```python
from build123d import *

# Parameters (mm, degrees)
SKETCH1_W           = 23
SKETCH1_H           = 12
BOSS_EXTRUDE1_DEPTH = 22
SKETCH2_W           = 32
SKETCH2_H           = 12
BOSS_EXTRUDE2_DEPTH = 2
CUT_EXTRUDE1_DEPTH  = 5
SKETCH3_W           = 23
SKETCH3_H           = 12
BOSS_EXTRUDE4_DEPTH = 4
BOSS_EXTRUDE5_DEPTH = 4
SKETCH6_R           = 2.5
SKETCH6_R_2         = 2.25
BOSS_EXTRUDE6_DEPTH = 2
CUT_EXTRUDE2_START  = -4
SKETCH7_R           = 2.25
CUT_EXTRUDE2_DEPTH  = 4
FILLET4_R           = 0.5
SKETCH8_R           = 2.25
BOSS_EXTRUDE7_DEPTH = 1
SKETCH9_R           = 0.75
BOSS_EXTRUDE8_DEPTH = 2


with BuildPart() as part:
    # Sketch1 → Boss-Extrude1 (new body)
    with BuildSketch(Plane(origin=(0, 0, 0), x_dir=(1, 0, 0), z_dir=(0, 1, 0))):
        Rectangle(SKETCH1_W, SKETCH1_H)
    extrude(amount=BOSS_EXTRUDE1_DEPTH)

    # Sketch2 → Boss-Extrude2 (add)
    with BuildSketch(Plane(origin=(0, 22, 0), x_dir=(1, 0, 0), z_dir=(0, 1, 0))):
        Rectangle(SKETCH2_W, SKETCH2_H)
    extrude(amount=BOSS_EXTRUDE2_DEPTH)

    # Sketch4 → Cut-Extrude1 (cut)
    with BuildSketch(Plane(origin=(0, 24, 0), x_dir=(1, 0, 0), z_dir=(0, 1, 0))):
        with BuildLine():
            Line((-16.63954717, 1), (-15.118033989, 1))
            ThreePointArc((-15.118033989, 1), (-12.5, 0), (-15.118033989, -1))
            Line((-15.118033989, -1), (-16.63954717, -1))
            Line((-16.63954717, -1), (-16.63954717, 1))
        make_face()
        with BuildLine():
            Line((15.118033989, 1), (17.121315796, 1))
            Line((17.121315796, 1), (17.121315796, -1))
            Line((17.121315796, -1), (15.118033989, -1))
            ThreePointArc((15.118033989, -1), (12.5, 0), (15.118033989, 1))
        make_face()
    extrude(amount=-CUT_EXTRUDE1_DEPTH, mode=Mode.SUBTRACT)

    # Sketch3 → Boss-Extrude4 (add)
    with BuildSketch(Plane(origin=(0, 24, 0), x_dir=(1, 0, 0), z_dir=(0, 1, 0))):
        Rectangle(SKETCH3_W, SKETCH3_H)
    extrude(amount=BOSS_EXTRUDE4_DEPTH)

    # Sketch5 → Boss-Extrude5 (add)
    with BuildSketch(Plane(origin=(0, 28, 0), x_dir=(1, 0, 0), z_dir=(0, 1, 0))):
        with BuildLine():
            ThreePointArc((-0.043232592, -2.296208273), (11.5, 0), (-0.043232592, 2.296208273))
            ThreePointArc((-0.043232592, 2.296208273), (-4.306483254, 0), (-0.043232592, -2.296208273))
        make_face()
    extrude(amount=BOSS_EXTRUDE5_DEPTH)

    # Sketch6 → Boss-Extrude6 (add)
    with BuildSketch(Plane(origin=(0, 32, 0), x_dir=(1, 0, 0), z_dir=(0, 1, 0))):
        with Locations(Location((5.5, 0, 0), (0, 0, 270))):
            Circle(SKETCH6_R)
        with Locations(Location((5.5, 0, 0), (0, 0, 270))):
            Circle(SKETCH6_R_2, mode=Mode.SUBTRACT)
    extrude(amount=BOSS_EXTRUDE6_DEPTH)

    # Sketch7 → Cut-Extrude2 (cut)
    with BuildSketch(Plane(origin=(0, 32, 0), x_dir=(1, 0, 0), z_dir=(0, 1, 0)).offset(CUT_EXTRUDE2_START)):
        with Locations(Location((5.5, 0, 0), (0, 0, 270))):
            Circle(SKETCH7_R)
    extrude(amount=CUT_EXTRUDE2_DEPTH, mode=Mode.SUBTRACT)

    # Fillet4
    fillet4_edges = [part.edges().sort_by_distance(p)[0] for p in [
        (5.5, 32, -2.5),
    ]]
    fillet(fillet4_edges, radius=FILLET4_R)

    # Sketch8 → Boss-Extrude7 (add)
    with BuildSketch(Plane(origin=(0, 0, -6), x_dir=(-1, 0, 0), z_dir=(0, 0, -1))):
        with Locations(Location((-5.5, 6, 0), (0, 0, 180))):
            Circle(SKETCH8_R)
    extrude(amount=BOSS_EXTRUDE7_DEPTH)

    # Sketch9 → Boss-Extrude8 (add)
    with BuildSketch(Plane(origin=(0, 0, -7), x_dir=(-1, 0, 0), z_dir=(0, 0, -1))):
        with Locations((-5.5, 6)):
            Circle(SKETCH9_R)
    extrude(amount=BOSS_EXTRUDE8_DEPTH)


solid = part.part
```
Work out the finished part from the listing and answer in its coordinate system (mm). A direction names the side the tool comes from. Coordinates: 2 decimals unless noted, no trailing zeros. Loops run counter-clockwise (first coordinate to the right, second up) from the corner with the lowest first, then second, coordinate; pieces in that order, holes last. Notation, with made-up numbers: (56, 28) - (101, 28) arc R17 ccw to (101, 40) - close; hole circle Ø9 at (88, 68.25). An arc over 180 degrees is marked (long way). Use a Markdown table: item, result.
Item 1: Find section C-C, the plane x = 1. Determine the outline of the cut face in (y, z).
Evaluation:
| item | result |
|---|---|
| outline | (0, -6) - (28, -6) - (28, -3.97) - (32, -3.97) - (32, 3.97) - (28, 3.97) - (28, 6) - (0, 6) - close |
Item 2: Find section A-A, the plane x = 14. Determine the outline of the cut face in (y, z).
Evaluation:
| item | result |
|---|---|
| outline | (22, -6) - (24, -6) - (24, -1.5) - (22, -1.5) - close; (22, 1.5) - (24, 1.5) - (24, 6) - (22, 6) - close |
Item 3: For faces 1 (the flat face through (11.5, 11, 0)), 2 (the flat face through (5, 5, -7)), 3 (the flat face through (-11.5, 26, 0)), determine the directions among +Z, -Z, +X, -X, +Y, -Y from which every point of the face is accessible in a straight line to the end or side of a thin tool.
Evaluation:
| item | result |
|---|---|
| face 1 | +Z, -Z, +X, -Y |
| face 2 | -Z |
| face 3 | +Z, -Z, -X, +Y |
Item 4: Find section B-B, the plane y = 6. Determine the outline of the cut face in (x, z).
Evaluation:
| item | result |
|---|---|
| outline | (-11.5, -6) - (3.25, -6) - (3.25, -7) - (4.75, -7) - (4.75, -9) - (6.25, -9) - (6.25, -7) - (7.75, -7) - (7.75, -6) - (11.5, -6) - (11.5, 6) - (-11.5, 6) - close |
Item 5: The mould has two halves that part along Z. Classify faces 4 (the cylindrical face through (11.496, 29.972, 0.231)), 5 (the flat face through (0, 14, 6)), 6 (the flat face through (11.5, 26, 0)), 7 (the cylindrical face through (-12.5, 23.01, -0.05)): +Z half, -Z half, draft (parallel to the pull), parting line (faces both ways), or undercut.
Evaluation:
| item | result |
|---|---|
| face 4 | parting line |
| face 5 | +Z half |
| face 6 | draft |
| face 7 | undercut |
Item 6: Consider probe 1 along X at (y, z) = (31.4, 0); probe 2 along Z at (x, y) = (14, 23.15); probe 3 along X at (y, z) = (23.2, 0). Determine where each line is inside the solid, lowest interval first. Write a range as from..to.
Evaluation:
| item | result |
|---|---|
| probe 1 | x = -4.31..3.25, 7.75..11.5 |
| probe 2 | z = -6..-1.5, 1.5..6 |
| probe 3 | x = -12.5..12.5 |
Item 7: Given pin 1 Ø6 at (y, z) = (12.5, 0) entering from -X; pin 2 Ø1.2 at (y, z) = (26, 2.5) entering from +X; pin 3 Ø1 at (x, y) = (-15.5, 23) entering from -Z, each flat-ended and moving along its own axis, determine where each tip first touches the part or whether it passes through.
Evaluation:
| item | result |
|---|---|
| pin 1 | stops at x = -11.5 |
| pin 2 | stops at x = 11.5 |
| pin 3 | stops at z = -6 |
Item 8: Find section D-D, the plane z = -5.25. Determine the outline of the cut face in (x, y).
Evaluation:
| item | result |
|---|---|
| outline | (-16, 22) - (-11.5, 22) - (-11.5, 0) - (11.5, 0) - (11.5, 22) - (16, 22) - (16, 24) - (11.5, 24) - (11.5, 28) - (8.4, 28) - (8.4, 32) - (2.6, 32) - (2.6, 28) - (-11.5, 28) - (-11.5, 24) - (-16, 24) - close |
